Verification items for the finished model (mm, model axes). A direction names the side the tool comes from. Give positions to 0.01 mm unless a question says otherwise; leave off trailing zeros. Loops run counter-clockwise (first coordinate to the right, second up) from the corner with the lowest first, then second, coordinate; pieces in that order, holes last. Notation, with made-up numbers: M -31,-37 L 14,-37 A23 cw 14,-27 Z; hole C 6,9 d7. An arc over 180 degrees is marked long. Answer in a Markdown table with one row per item.
```python
from build123d import *

# Parameters (mm, degrees)
F0_W      = 46
F0_H      = 80
F1_DEPTH  = 25
F4_DEPTH  = 60
F5_DEPTH  = 46
F8_DEPTH  = 3.5
F10_DEPTH = 0.4


with BuildPart() as f1:
    # F0 (on Front) → F1 (new body)
    with BuildSketch(Plane.XZ):
        with Locations((-12.4670048244, -31.5567021806)):
            Rectangle(F0_W, F0_H)
    extrude(amount=F1_DEPTH)

    # F3 (on face) → F4 (join)
    with BuildSketch(Plane.XY.offset(8.4432978194)):
        Polygon((10.5329951756, -25), (10.5329951756, 0), (-1.4670048244, 0), (-1.4670048244, -5), (5.5329951756, -5), (5.5329951756, -20), (-30.4670048244, -20), (-30.4670048244, -5), (-23.4670048244, -5), (-23.4670048244, 0), (-35.4670048244, 0), (-35.4670048244, -25), align=None)
    extrude(amount=F4_DEPTH)

    # F2 (on face) → F5 (join)
    with BuildSketch(Plane(origin=(-35.4670048244, 0, 0), x_dir=(0, -1, 0), z_dir=(-1, 0, 0))):
        Polygon((-100, -71.5567021806), (0, -71.5567021806), (0, -67.5567021806), (-70, -67.5567021806), (-100, -67.5567021806), align=None)
        Polygon((25, -67.5567021806), (25, -71.5567021806), (145, -71.5567021806), (145, -67.5567021806), (115, -67.5567021806), align=None)
    extrude(amount=-F5_DEPTH)

    # F7 (on offset) → F8 (join, symmetric)
    with BuildSketch(Plane(origin=(-12.4670048244, 0, 0), x_dir=(0, -1, 0), z_dir=(-1, 0, 0))):
        Polygon((0, -67.5567021806), (0, 2.4432978194), (-70, -67.5567021806), align=None)
        Polygon((25, 2.4432978194), (25, -67.5567021806), (115, -67.5567021806), align=None)
    extrude(amount=F8_DEPTH, both=True)

    # F10 (add, through all): a face of the model
    f10_faces = [f1.faces().sort_by_distance(p)[0] for p in [
        (-12.4670048244, -10.8076923077, 8.4432978194),
    ]]
    extrude(f10_faces, amount=F10_DEPTH)


solid = f1.part
```
Item 1: Sectioned sample at A-A (z = 33). Record the cut outline in (x, y), and give its area (3 significant figures).
Reported:
| item | result |
|---|---|
| outline | M -35.47,-25 L 10.53,-25 L 10.53,0 L -1.47,0 L -1.47,-5 L 5.53,-5 L 5.53,-20 L -30.47,-20 L -30.47,-5 L -23.47,-5 L -23.47,0 L -35.47,0 Z |
| area | 500 mm^2 |
Item 2: Go/stop test with flat-tipped pins: pin 1 (21 mm diameter, centred on y = 28.5, z = -43.5, fed in from +X); pin 2 (5 mm diameter, centred on x = -16.5, y = -32, fed in from +Z); pin 3 (5.5 mm diameter, centred on x = 0.5, z = 26, fed in from -Y). Record where each tip stops, or that it passes through.
Reported:
| item | result |
|---|---|
| pin 1 | stops at x = -8.97 |
| pin 2 | stops at z = -1.1 |
| pin 3 | stops at y = -25 |
Item 3: Scan lines: L1, parallel to Y at x = -0.5, z = 15.5; L2, parallel to Z at x = -31.5, y = 22; L3, parallel to Y at x = -17.5, z = 33. Record each from-to range of solid material in increasing order. Write a range as [from, to].
Reported:
| item | result |
|---|---|
| L1 | y = [-25, -20], [-5, 0] |
| L2 | z = [-71.56, -67.56] |
| L3 | y = [-25, -20] |
Item 4: Sectioned sample at B-B (x = -13.5). Record the cut outline in (y, z).
Reported:
| item | result |
|---|---|
| outline | M -145,-71.56 L 100,-71.56 L 100,-67.56 L 70,-67.56 L 0,2.44 L 0,8.84 L -20,8.84 L -20,68.44 L -25,68.44 L -25,2.44 L -115,-67.56 L -145,-67.56 Z |
Item 5: Release check for a two-part mould opening along X. For faces 1 (the flat face through (-35.467, -13, -22)), 2 (the flat face through (-8.967, 20, -48)), 3 (the flat face through (-12, -20, 38)) record: released by +X, released by -X, zero draft, split by the parting line, or undercut.
Reported:
| item | result |
|---|---|
| face 1 | released by -X |
| face 2 | released by +X |
| face 3 | undercut |
Item 6: Sectioned sample at C-C (y = -9). Record the cut outline in (x, z).
Reported:
| item | result |
|---|---|
| outline | M -35.47,-71.56 L 10.53,-71.56 L 10.53,68.44 L 5.53,68.44 L 5.53,8.84 L -30.47,8.84 L -30.47,68.44 L -35.47,68.44 Z |
Item 7: Sectioned sample at D-D (y = -59.5). Record the cut outline in (x, z).
Reported:
| item | result |
|---|---|
| outline | M -35.47,-71.56 L 10.53,-71.56 L 10.53,-67.56 L -8.97,-67.56 L -8.97,-24.39 L -15.97,-24.39 L -15.97,-67.56 L -35.47,-67.56 Z |
Item 8: Tool access check on faces 4 (the flat face through (-18, 49, -67.557)), 5 (the flat face through (-15.967, 20, -48)), 6 (the flat face through (-30.467, -13, 38)), 7 (the flat face through (-15.967, -49, -48)), 8 (the flat face through (-8.967, -49, -48)). Record the directions out of +Z, -Z, +X, -X, +Y, -Y that give a thin tool (end or side, any length) a straight path to the whole face; none if there is none.
Reported:
| item | result |
|---|---|
| face 4 | +Z, +Y |
| face 5 | +Z, -X, +Y |
| face 6 | +Z |
| face 7 | +Z, -X, -Y |
| face 8 | +Z, +X, -Y |
